from build123d import *

# Parameters (mm, degrees)
SKETCH1_R           = 1.575
BOSS_EXTRUDE1_DEPTH = 1.6


with BuildPart() as part:
    # Sketch1 → Boss-Extrude1 (new body)
    with BuildSketch(Plane(origin=(0, 0, 0), x_dir=(1, 0, 0), z_dir=(0, 1, 0))):
        with BuildLine():
            Line((-50, 24.125), (-32.915475947, 24.125))
            ThreePointArc((-32.915475947, 24.125), (-31.68372891, 24.449500233), (-30.771743633, 25.338760611))
            Line((-30.771743633, 25.338760611), (-30.728256367, 25.411239389))
            ThreePointArc((-30.728256367, 25.411239389), (-29.81627109, 26.300499767), (-28.584524053, 26.625))
            Line((-28.584524053, 26.625), (-26.415475947, 26.625))
            ThreePointArc((-26.415475947, 26.625), (-25.18372891, 26.300499767), (-24.271743633, 25.411239389))
            Line((-24.271743633, 25.411239389), (-24.228256367, 25.338760611))
            ThreePointArc((-24.228256367, 25.338760611), (-23.31627109, 24.449500233), (-22.084524053, 24.125))
            Line((-22.084524053, 24.125), (-7.915475947, 24.125))
            ThreePointArc((-7.915475947, 24.125), (-6.68372891, 24.449500233), (-5.771743633, 25.338760611))
            Line((-5.771743633, 25.338760611), (-5.728256367, 25.411239389))
            ThreePointArc((-5.728256367, 25.411239389), (-4.81627109, 26.300499767), (-3.584524053, 26.625))
            Line((-3.584524053, 26.625), (-1.415475947, 26.625))
            ThreePointArc((-1.415475947, 26.625), (-0.18372891, 26.300499767), (0.728256367, 25.411239389))
            Line((0.728256367, 25.411239389), (0.771743633, 25.338760611))
            ThreePointArc((0.771743633, 25.338760611), (1.68372891, 24.449500233), (2.915475947, 24.125))
            Line((2.915475947, 24.125), (17.084524053, 24.125))
            ThreePointArc((17.084524053, 24.125), (18.31627109, 24.449500233), (19.228256367, 25.338760611))
            Line((19.228256367, 25.338760611), (19.271743633, 25.411239389))
            ThreePointArc((19.271743633, 25.411239389), (20.18372891, 26.300499767), (21.415475947, 26.625))
            Line((21.415475947, 26.625), (23.584524053, 26.625))
            ThreePointArc((23.584524053, 26.625), (24.81627109, 26.300499767), (25.728256367, 25.411239389))
            Line((25.728256367, 25.411239389), (25.771743633, 25.338760611))
            ThreePointArc((25.771743633, 25.338760611), (26.68372891, 24.449500233), (27.915475947, 24.125))
            Line((27.915475947, 24.125), (50, 24.125))
            Line((50, 24.125), (50, -24.125))
            Line((50, -24.125), (27.915475947, -24.125))
            ThreePointArc((27.915475947, -24.125), (26.68372891, -24.449500233), (25.771743633, -25.338760611))
            Line((25.771743633, -25.338760611), (25.728256367, -25.411239389))
            ThreePointArc((25.728256367, -25.411239389), (24.81627109, -26.300499767), (23.584524053, -26.625))
            Line((23.584524053, -26.625), (21.415475947, -26.625))
            ThreePointArc((21.415475947, -26.625), (20.18372891, -26.300499767), (19.271743633, -25.411239389))
            Line((19.271743633, -25.411239389), (19.228256367, -25.338760611))
            ThreePointArc((19.228256367, -25.338760611), (18.31627109, -24.449500233), (17.084524053, -24.125))
            Line((17.084524053, -24.125), (2.915475947, -24.125))
            ThreePointArc((2.915475947, -24.125), (1.68372891, -24.449500233), (0.771743633, -25.338760611))
            Line((0.771743633, -25.338760611), (0.728256367, -25.411239389))
            ThreePointArc((0.728256367, -25.411239389), (-0.18372891, -26.300499767), (-1.415475947, -26.625))
            Line((-1.415475947, -26.625), (-3.584524053, -26.625))
            ThreePointArc((-3.584524053, -26.625), (-4.81627109, -26.300499767), (-5.728256367, -25.411239389))
            Line((-5.728256367, -25.411239389), (-5.771743633, -25.338760611))
            ThreePointArc((-5.771743633, -25.338760611), (-6.68372891, -24.449500233), (-7.915475947, -24.125))
            Line((-7.915475947, -24.125), (-22.084524053, -24.125))
            ThreePointArc((-22.084524053, -24.125), (-23.31627109, -24.449500233), (-24.228256367, -25.338760611))
            Line((-24.228256367, -25.338760611), (-24.271743633, -25.411239389))
            ThreePointArc((-24.271743633, -25.411239389), (-25.18372891, -26.300499767), (-26.415475947, -26.625))
            Line((-26.415475947, -26.625), (-28.584524053, -26.625))
            ThreePointArc((-28.584524053, -26.625), (-29.81627109, -26.300499767), (-30.728256367, -25.411239389))
            Line((-30.728256367, -25.411239389), (-30.771743633, -25.338760611))
            ThreePointArc((-30.771743633, -25.338760611), (-31.68372891, -24.449500233), (-32.915475947, -24.125))
            Line((-32.915475947, -24.125), (-50, -24.125))
            Line((-50, -24.125), (-50, 24.125))
        make_face()
        with Locations(Location((-27.5, -22.375, 0), (0, 0, 270))):
            Circle(SKETCH1_R, mode=Mode.SUBTRACT)
        with Locations(Location((-27.5, 22.375, 0), (0, 0, 90))):
            Circle(SKETCH1_R, mode=Mode.SUBTRACT)
        with Locations(Location((-2.5, 22.375, 0), (0, 0, 90))):
            Circle(SKETCH1_R, mode=Mode.SUBTRACT)
        with Locations(Location((-2.5, -22.375, 0), (0, 0, 270))):
            Circle(SKETCH1_R, mode=Mode.SUBTRACT)
        with Locations(Location((22.5, 22.375, 0), (0, 0, 90))):
            Circle(SKETCH1_R, mode=Mode.SUBTRACT)
        with Locations(Location((22.5, -22.375, 0), (0, 0, 270))):
            Circle(SKETCH1_R, mode=Mode.SUBTRACT)
    extrude(amount=BOSS_EXTRUDE1_DEPTH)


solid = part.part
CAD build for the part. Positions are in the model's coordinates, mm. Coordinates: 2 decimals unless noted, no trailing zeros. Loops run counter-clockwise (first coordinate to the right, second up) from the corner with the lowest first, then second, coordinate; pieces in that order, holes last. Notation, with made-up numbers: (61.25, -13) -> (97.25, -13) arc R11 cw to (97.25, 3) -> close; hole circle Ø9 at (33, 78). An arc over 180 degrees is marked (long way). One line per item, written item: value.
1. Slice it at A-A on x = -2.5. Write the cut outline in (y, z) (3 decimals).
Answers:
outline: (0, -26.625) -> (1.6, -26.625) -> (1.6, -23.95) -> (0, -23.95) -> close; (0, -20.8) -> (1.6, -20.8) -> (1.6, 20.8) -> (0, 20.8) -> close; (0, 23.95) -> (1.6, 23.95) -> (1.6, 26.625) -> (0, 26.625) -> close
2. Slice it at B-B on z = -23. Write the cut outline in (x, y), and give its area (3 significant figures).
Answers:
outline: (-50, 0) -> (-28.95, 0) -> (-28.95, 1.6) -> (-50, 1.6) -> close; (-26.05, 0) -> (-3.95, 0) -> (-3.95, 1.6) -> (-26.05, 1.6) -> close; (-1.05, 0) -> (21.05, 0) -> (21.05, 1.6) -> (-1.05, 1.6) -> close; (23.95, 0) -> (50, 0) -> (50, 1.6) -> (23.95, 1.6) -> close
area: 146 mm^2
3. Slice it at D-D on x = -43. Write the cut outline in (y, z) (3 decimals), and give its area (3 significant figures).
Answers:
outline: (0, -24.125) -> (1.6, -24.125) -> (1.6, 24.125) -> (0, 24.125) -> close
area: 77.2 mm^2
4. Flat gauge pins, fed straight in: P1, Ø0.8, axis at x = 40.5, y = 1, coming from the +Z side (3 decimals); P2, Ø0.8, axis at x = -15.5, y = 0.5, coming from the -Z side (3 decimals). Where does each tip first touch, or does it go through?
Answers:
P1: stops at z = 24.125
P2: stops at z = -24.125
5. Pull direction X, two halves, no side cores. Call faces 1 (the face through (1, 1.6, 0)), 2 (the face through (20.962, 0.789, 22.034)): pulls with the +X half, pulls with the -X half, needs draft (parallel to the pull), parting line crosses it, or undercut.
Answers:
face 1: needs draft
face 2: undercut
6. Drill centre lines: line 1 (X direction, y = 0.1, z = -21.5); line 2 (Z direction, x = -16.5, y = 0.7) (3 decimals); line 3 (Z direction, x = -28, y = 1.25) (3 decimals). Where is each one in solid material? Low to high. Write a range as [from, to].
Answers:
line 1: x = [-50, -28.81], [-26.19, -3.81], [-1.19, 21.19], [23.81, 50]
line 2: z = [-24.125, 24.125]
line 3: z = [-26.625, -23.869], [-20.881, 20.881], [23.869, 26.625]
7. Slice it at C-C on y = 0.5. Give the number of separate pieces and of enclosed holes in the cut face, and give its area (3 significant figures).
Answers:
separate pieces: 1
enclosed holes: 6
area: 4,880 mm^2
